Source: CAD feature listing. Evaluate the final solid. Frame: model axes, mm. Face numbers are marked on the shaded views. A direction names the side the tool comes from. Give positions to 0.01 mm unless a question says otherwise; leave off trailing zeros. Order: outer loops, then holes, each group sorted by start corner. A loop starts at its lowest first (then second) coordinate and runs counter-clockwise, first axis right, second up. Notation, with made-up numbers: M 56,31.25 L 81,31.25 A26 ccw 81,54.25 Z; hole C 50.5,19.5 d2. An arc over 180 degrees is marked long. One line per question, with ' | ' between items. Start each with the question number.
from build123d import *

# Parameters (mm, degrees)
SKETCH_1_W          = 65
SKETCH_1_H          = 25
EXTRUDE_1_DEPTH     = 4
SKETCH_2_W          = 15
SKETCH_2_H          = 25
EXTRUDE_2_DEPTH     = 13
SKETCH_3_R          = 2.5
SKETCH_3_R_2        = 4
CUT_EXTRUDE_1_DEPTH = 39.74919354
SKETCH_5_W          = 15
SKETCH_5_H          = 4
EXTRUDE_3_DEPTH     = 6
SKETCH_6_R          = 1.25
CUT_EXTRUDE_3_DEPTH = 40.59166579
FILLET_2_R          = 3
CUT_EXTRUDE_4_DEPTH = 49.023431781


with BuildPart() as part:
    # 草图1 → 凸台-拉伸1 (new body)
    with BuildSketch(Plane(origin=(0, 0, 0), x_dir=(1, 0, 0), z_dir=(0, 1, 0))):
        Rectangle(SKETCH_1_W, SKETCH_1_H)
    extrude(amount=EXTRUDE_1_DEPTH)

    # 草图2 → 凸台-拉伸2 (add)
    with BuildSketch(Plane(origin=(0, 4, 0), x_dir=(1, 0, 0), z_dir=(0, 1, 0))):
        Rectangle(SKETCH_2_W, SKETCH_2_H)
    extrude(amount=EXTRUDE_2_DEPTH)

    # 草图3 → 切除-拉伸1 (cut, through all)
    with BuildSketch(Plane.XZ):
        with Locations(Location((0, -7.5, 0), (0, 0, 270))):
            Circle(SKETCH_3_R)
        with Locations(Location((0, 7.5, 0), (0, 0, 90))):
            Circle(SKETCH_3_R)
        with Locations(Location((-22, 0, 0), (0, 0, 270))):
            Circle(SKETCH_3_R_2)
        with Locations(Location((22, 0, 0), (0, 0, 90))):
            Circle(SKETCH_3_R_2)
    extrude(amount=-CUT_EXTRUDE_1_DEPTH, mode=Mode.SUBTRACT)

    # 草图5 → 凸台-拉伸3 (add)
    with BuildSketch(Plane.XY.offset(12.5)):
        with Locations((0, 6)):
            Rectangle(SKETCH_5_W, SKETCH_5_H)
    extrude_3 = extrude(amount=EXTRUDE_3_DEPTH)

    # 草图6 → 切除-拉伸3 (cut, through all)
    with BuildSketch(Plane.XZ.offset(-4)):
        with Locations(Location((-4.5, 15.5, 0), (0, 0, 270))):
            Circle(SKETCH_6_R)
        with Locations(Location((4.5, 15.5, 0), (0, 0, 270))):
            Circle(SKETCH_6_R)
    cut_extrude_3 = extrude(amount=-CUT_EXTRUDE_3_DEPTH, mode=Mode.SUBTRACT)

    # 镜向2: 凸台-拉伸3, 切除-拉伸3 across plane
    add(extrude_3.mirror(Plane.XY))
    add(cut_extrude_3.mirror(Plane.XY), mode=Mode.SUBTRACT)

    # 圆角2
    fillet_2_edges = [part.edges().sort_by_distance(p)[0] for p in [
        (-7.5, 6, 18.5),
        (7.5, 6, 18.5),
        (-7.5, 6, -18.5),
        (7.5, 6, -18.5),
    ]]
    fillet(fillet_2_edges, radius=FILLET_2_R)

    # 草图7 → 切除-拉伸4 (cut, through all)
    with BuildSketch(Plane(origin=(0, 0, -12.5), x_dir=(-1, 0, 0), z_dir=(0, 0, -1))):
        Polygon((32.5, 4), (7.5, 4), (-7.5, 4), (-32.5, 4), (-32.5, 0), (32.5, 0), align=None)
    extrude(amount=-CUT_EXTRUDE_4_DEPTH, mode=Mode.SUBTRACT)


solid = part.part
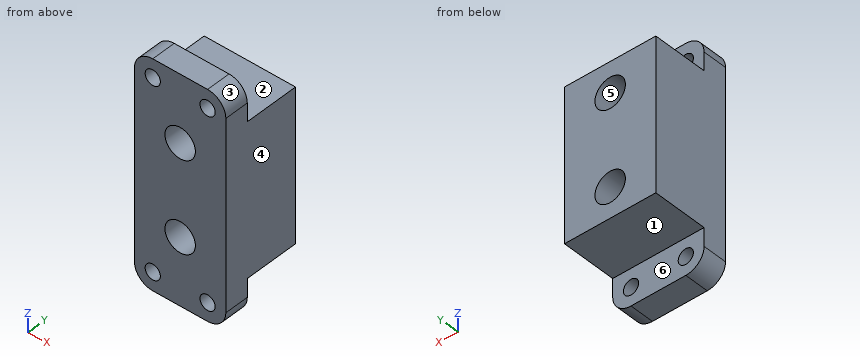
Item 1: Mould query, pull axis X, two halves, no side actions, for the marked faces 4, 5 and 6. Classes: pulls with the +X half, pulls with the -X half, needs draft (parallel to the pull), parting line crosses it, or undercut.
Item 2: Cut plane A-A on z = -9.5. Return the cut outline in (x, y), and give its area (3 significant figures).
Item 3: Cut plane B-B on x = -3.75. Return the cut outline in (y, z), and give its area (3 significant figures).
Item 4: Pin query (flat end, axial travel): pin 1 Ø1.8 at (x, z) = (-3.5, 15) entering from +Y; pin 2 Ø4 at (x, z) = (0, 7.5) entering from -Y; pin 3 Ø1 at (x, y) = (-5.5, 5.5) entering from -Z; pin 4 Ø7 at (x, y) = (-0.5, 13.5) entering from +Z. Return the tip coordinate at first contact, or that it passes through.
Item 5: Reachability of the marked faces 1, 2 and 3 from +Z, -Z, +X, -X, +Y, -Y: full face, straight path, thin tool, end or side. Return the list, or none.
Item 6: Cut plane D-D on z = 7.5. Return the cut outline in (x, y), and give its area (3 significant figures).
Item 7: Cut plane C-C on y = 15. Return the cut outline in (x, z), and give its area (3 significant figures).
Item 8: Line query: line 1 (X direction, y = 5.9, z = 15.5); line 2 (X direction, y = 11.5, z = -7.5); line 3 (Y direction, x = 3.75, z = -14). Output: solid intervals per line, ascending.
Results are:
1) face 4: pulls with the +X half | face 5: undercut | face 6: needs draft
2) outline: M -7.5,4 L -1.5,4 L -1.5,17 L -7.5,17 Z; M 1.5,4 L 7.5,4 L 7.5,17 L 1.5,17 Z | area: 156 mm2
3) outline: M 4,-18.5 L 8,-18.5 L 8,-16.5 L 4,-16.5 Z; M 4,-14.5 L 8,-14.5 L 8,-12.5 L 17,-12.5 L 17,12.5 L 8,12.5 L 8,14.5 L 4,14.5 Z; M 4,16.5 L 8,16.5 L 8,18.5 L 4,18.5 Z | area: 357 mm2
4) pin 1: stops at y = 8 | pin 2: passes through | pin 3: stops at z = -18.46 | pin 4: stops at z = 12.5
5) face 1: -Z, +X, -X, +Y | face 2: +Z, +X, -X, +Y | face 3: +Z, +X, +Y, -Y
6) outline: M -7.5,4 L -2.5,4 L -2.5,17 L -7.5,17 Z; M 2.5,4 L 7.5,4 L 7.5,17 L 2.5,17 Z | area: 130 mm2
7) outline: M -7.5,-12.5 L 7.5,-12.5 L 7.5,12.5 L -7.5,12.5 Z; hole C 0,-7.5 d5; hole C 0,7.5 d5 | area: 336 mm2
8) line 1: x = -7.5 to -5.75, -3.25 to 3.25, 5.75 to 7.5 | line 2: x = -7.5 to -2.5, 2.5 to 7.5 | line 3: y = 4 to 8
